The model under review builds one solid part; all positions refer to its coordinate system, in mm. Face numbers are marked on the shaded views. Round coordinates to 2 decimals unless told otherwise and drop trailing zeros. Loops run counter-clockwise (first coordinate to the right, second up) from the corner with the lowest first, then second, coordinate; pieces in that order, holes last. Notation, with made-up numbers: M 53,-26 L 61,-26 A12 ccw 61,-13 Z; hole C 89.5,32.25 d3. An arc over 180 degrees is marked long. Answer as a JSON object with one key per item and string values. Group by question number.
Item 1: The part is to be moulded in two halves that separate along Y. For the marked faces 1 and 2, say which applies: +Y half, -Y half, draft (parallel to the pull), parting line (faces both ways), or undercut.
Item 2: Consider section B-B (z = -17.5). Give the boundary of the cut face in (x, y), and give its area (3 significant figures).
Item 3: Consider section A-A (y = 0). Give the boundary of the cut face in (x, z), and give its area (3 significant figures).
Item 4: Consider section C-C (x = 23). Give the boundary of the cut face in (y, z).
Item 5: Insertion check: P1, Ø4, axis at x = 16, y = 5, coming from the -Z side; P2, Ø12, axis at y = -24, z = -17.5, coming from the +X side; P3, Ø2, axis at x = 28.5, y = 2, coming from the +Z side; P4, Ø2, axis at x = -4.5, z = -24, coming from the -Y side. Each pin has a flat end and moves straight along its axis. Give the tip position at first contact, or say it passes through.
Item 6: To check wall thickness, follow line 1 (Z direction, x = 23.5, y = 0); line 2 (Y direction, x = 15.5, z = -19); line 3 (Y direction, x = 28.5, z = -16). State the ranges of each line that lie inside material, in increasing order.
```python
from build123d import *

# Parameters (mm, degrees)
SWEEP1_PITCH       = 0.704426667
SWEEP1_HEIGHT      = 1.3208
SWEEP1_RADIUS      = 28.5496
SWEEP1_START_ANGLE = 180
SKETCH3_W          = 0.6604
SKETCH3_H          = 5.08
CUT_EXTRUDE4_DEPTH = 0.682414
CUT_EXTRUDE3_DEPTH = 0.682398


with BuildPart() as part:
    # Sweep1: sweep along a helix
    with BuildLine() as sweep1_path:
        add(Helix(SWEEP1_PITCH, SWEEP1_HEIGHT, SWEEP1_RADIUS, center=(0, 0, 0), direction=(1, 0, 0), mode=Mode.PRIVATE).rotate(Axis((0, 0, 0), (1, 0, 0)), SWEEP1_START_ANGLE))
    # Sketch3 → Sweep1 (sweep)
    with BuildSketch(Plane(origin=(0, 0, 0), x_dir=(1, 0, 0), z_dir=(0, 1, 0))):
        with Locations((0.3302, 31.0896)):
            Rectangle(SKETCH3_W, SKETCH3_H)
    sweep(path=sweep1_path.line, is_frenet=True)

    # Sketch8 → Cut-Extrude4 (cut)
    with BuildSketch(Plane(origin=(0, 0, 0), x_dir=(0, 0, -1), z_dir=(1, 0, 0))):
        with BuildLine():
            Line((30.242933333, 0), (33.6296, 0))
            ThreePointArc((33.6296, 0), (33.118690811, 5.839718756), (31.60148696, 11.502000612))
            ThreePointArc((31.60148696, 11.502000612), (30.583748126, 5.790977595), (30.242933333, 0))
        make_face()
    extrude(amount=CUT_EXTRUDE4_DEPTH, mode=Mode.SUBTRACT)

    # Sketch7 → Cut-Extrude3 (cut)
    with BuildSketch(Plane(origin=(1.980679935, 0, 0), x_dir=(0, 0, -1), z_dir=(1, 0, 0))):
        with BuildLine():
            Line((21.384984059, -21.384982427), (23.779719052, -23.779717365))
            ThreePointArc((23.779719052, -23.779717365), (19.289146911, -27.547755038), (14.212483755, -30.478768047))
            ThreePointArc((14.212483755, -30.478768047), (17.531136878, -25.720814646), (21.384984059, -21.384982427))
        make_face()
    extrude(amount=-CUT_EXTRUDE3_DEPTH, mode=Mode.SUBTRACT)


with BuildPart() as body_2:
    # Sketch2 → Revolve1 (revolve)
    with BuildSketch(Plane.XY):
        Polygon((-9.931660032, -31.75), (-9.931660032, -35.5092), (33.756339968, -35.5092), (33.756339968, -31.75), (2.082539968, -31.75), (2.082539968, -33.6296), (-0.101860032, -33.6296), (-0.101860032, -31.75), align=None)
    revolve(axis=Axis((33.756339968, 0, 0), (-1, 0, 0)))


solid = body_2.part
```
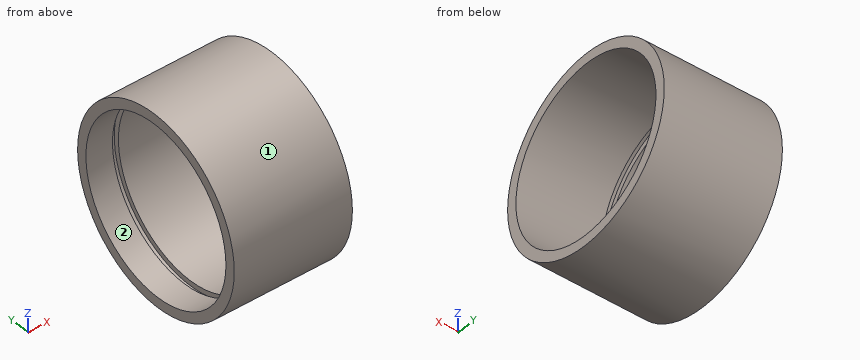
Geometry results:
{
 "1": {"face 1": "parting line", "face 2": "undercut"},
 "2": {"outline": "M -9.93,-30.9 L 33.76,-30.9 L 33.76,-26.49 L 2.08,-26.49 L 2.08,-28.72 L -0.1,-28.72 L -0.1,-26.49 L -9.93,-26.49 Z; M -9.93,26.49 L -0.1,26.49 L -0.1,28.72 L 2.08,28.72 L 2.08,26.49 L 33.76,26.49 L 33.76,30.9 L -9.93,30.9 Z", "area": "375 mm^2"},
 "3": {"outline": "M -9.93,-35.51 L 33.76,-35.51 L 33.76,-31.75 L 2.08,-31.75 L 2.08,-33.63 L -0.1,-33.63 L -0.1,-31.75 L -9.93,-31.75 Z; M -9.93,31.75 L -0.1,31.75 L -0.1,33.63 L 2.08,33.63 L 2.08,31.75 L 33.76,31.75 L 33.76,35.51 L -9.93,35.51 Z", "area": "320 mm^2"},
 "4": {"outline": "C 0,0 d71.02; hole C 0,0 d63.5"},
 "5": {"P1": "stops at z = -35.38", "P2": "stops at x = 33.76", "P3": "stops at z = 35.5", "P4": "stops at y = -27.05"},
 "6": {"line 1": "z = -35.51 to -31.75, 31.75 to 35.51", "line 2": "y = -30 to -25.44, 25.44 to 30", "line 3": "y = -31.7 to -27.42, 27.42 to 31.7"}
}
